Study the drawing (mm; zero at the part's minimum x, y, z) and answer. Round coordinates to 2 decimals unless told otherwise and drop trailing zeros. Loops run counter-clockwise (first coordinate to the right, second up) from the corner with the lowest first, then second, coordinate; pieces in that order, holes last. Notation, with made-up numbers: (75.25, 32) -> (101.25, 32) arc R12 cw to (101.25, 48) -> close; hole circle Ø3 at (21.25, -28.5). An arc over 180 degrees is marked (long way). Use one line per item in the form item = value.
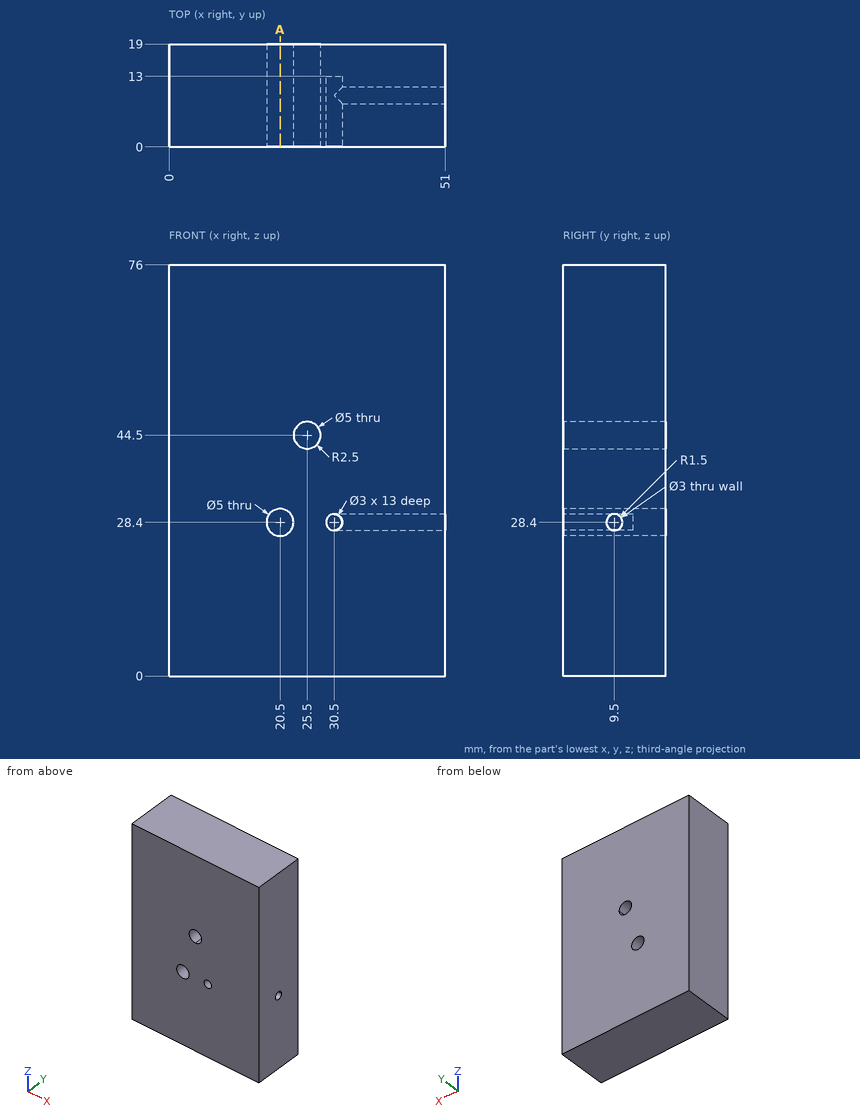
(1) Consider L1, parallel to Z at x = 25.5, y = 13.5; L2, parallel to Z at x = 30.5, y = 7.25; L3, parallel to X at y = 10.5, z = 44.5. Determine where each line is inside the solid, lowest interval first.
Completed:
L1 = 0 to 42, 47 to 76
L2 = 0 to 26.9, 29.9 to 76
L3 = 0 to 23, 28 to 51
(2) Find section A-A, the plane x = 20.5. Write down the section's boundary in (y, z).
Completed:
outline = (0, 0) -> (19, 0) -> (19, 25.9) -> (0, 25.9) -> close; (0, 30.9) -> (19, 30.9) -> (19, 76) -> (0, 76) -> close
(3) Given P1, Ø0.9, axis at x = 30.5, z = 27.5, coming from the -Y side, flat-ended and moving along its own axis, determine where the tip first touches the part or whether it passes through.
Completed:
P1 = 13
